Could you check a few things on this model? Use its own coordinates, in mm. A direction names the side the tool comes from. Round coordinates to 2 decimals unless told otherwise and drop trailing zeros. Write each loop counter-clockwise with the first axis right and the second up, starting at its lowest first coordinate (ties: lowest second). Pieces come first, ordered by that corner, then holes. Notation, with made-up numbers: (-7.5, 0) -> (6.5, 0) arc R18 cw to (6.5, 11) -> close; hole circle Ø4 at (-30.5, 19.5). An arc over 180 degrees is marked (long way). Answer as CSV lines item,"result". Start each with the question number.
Q1. Imagine slicing it at C-C on y = -16. Give the number of separate pieces and of enclosed holes in the cut face, and give its area (3 significant figures).
Q2. If we mould it in two halves opening along X, with no side actions, what happens to faces 4 (the cylindrical face through (68.496, -14.84, 117.029)), 5 (the flat face through (0, 96, 8)), 6 (the flat face through (55, -29, 60))? For each: pulls with the +X half, pulls with the -X half, needs draft (parallel to the pull), parting line crosses it, or undercut.
Q3. Imagine slicing it at B-B on z = 21.5. Please give me the cut outline in (x, y), and give its area (3 significant figures).
Q4. For faces 1 (the cylindrical face through (44.74, 91.85, 3.94)), 2 (the cylindrical face through (-57.093, -35.291, 4.094)), 3 (the flat face through (62.827, 24.837, 3.857)), which set-ups out of +Z, -Z, +X, -X, +Y, -Y let a thin tool reach every point of the face, with its end or its side?
Q5. Imagine slicing it at A-A on x = -5. Please give me the cut outline in (y, z), and give its area (3 significant figures).
Q6. Will these pins go through, and if not, where does the flat tip stop? pin 1 Ø8 at (x, z) = (-53, 50) entering from -Y; pin 2 Ø12 at (x, y) = (-43.5, 38.5) entering from -Z.
from build123d import *

# Parameters (mm, degrees)
F1_DEPTH      = 8
F3_DEPTH      = 70
F3_DEPTH_BACK = 70
F4_W          = 110
F4_H          = 115
F4_R          = 2
F5_DEPTH      = 10.5877977107
F6_R          = 5
F7_R          = 5


with BuildPart() as f1:
    # F0 (on Top) → F1 (new body)
    with BuildSketch(Plane.XY):
        with BuildLine():
            Line((-55.4502481405, 98.6044170713), (-70, -46.8931015238))
            Line((-70, -46.8931015238), (70, -46.8931015238))
            Line((70, -46.8931015238), (55.4502481405, 98.6044170713))
            ThreePointArc((55.4502481405, 98.6044170713), (53.8300887932, 101.8141611439), (50.4750621894, 103.1068984762))
            Line((50.4750621894, 103.1068984762), (-50.4750621894, 103.1068984762))
            ThreePointArc((-50.4750621894, 103.1068984762), (-53.8300887932, 101.8141611439), (-55.4502481405, 98.6044170713))
        make_face()
        with BuildLine():
            Line((-41.4251865683, 93.1068984762), (41.4251865683, 93.1068984762))
            ThreePointArc((41.4251865683, 93.1068984762), (44.7802131721, 91.8141611439), (46.4003725194, 88.6044170713))
            Line((46.4003725194, 88.6044170713), (58.4003725194, -31.3955829287))
            ThreePointArc((58.4003725194, -31.3955829287), (57.1324492361, -35.2481281276), (53.4251865683, -36.8931015238))
            Line((53.4251865683, -36.8931015238), (-53.4251865683, -36.8931015238))
            ThreePointArc((-53.4251865683, -36.8931015238), (-57.1324492361, -35.2481281276), (-58.4003725194, -31.3955829287))
            Line((-58.4003725194, -31.3955829287), (-46.4003725194, 88.6044170713))
            ThreePointArc((-46.4003725194, 88.6044170713), (-44.7802131721, 91.8141611439), (-41.4251865683, 93.1068984762))
        make_face(mode=Mode.SUBTRACT)
    extrude(amount=F1_DEPTH)

    # F2 (on Right) → F3 (join, two sides)
    with BuildSketch(Plane.YZ) as f3_sk:
        Polygon((-18.3058557984, 119.3901673481), (-46.8931015238, 8), (-38.633844698, 8), (-35.4294686048, 20.4858474544), (-10.5569745916, 117.4014893846), align=None)
    extrude(amount=F3_DEPTH)
    extrude(f3_sk.sketch, amount=-F3_DEPTH_BACK)

    # F4 (on face) → F5 (cut, through all)
    with BuildSketch(Plane(origin=(0, -45.9216252544, 11.7853560733), x_dir=(1, 0, 0), z_dir=(0, -0.9686101509, 0.2485847454))):
        with Locations((0, 53.5919715017)):
            Rectangle(F4_W, F4_H)
        with Locations((-62.5, 101.0919715017)):
            Circle(F4_R)
        with Locations((-62.5, 36.0919715017)):
            Circle(F4_R)
        with Locations((62.5, 36.0919715017)):
            Circle(F4_R)
        with Locations((62.5, 101.0919715017)):
            Circle(F4_R)
    extrude(amount=-F5_DEPTH, mode=Mode.SUBTRACT)

    # F6
    f6_edges = [f1.edges().sort_by_distance(p)[0] for p in [
        (-70, -14.431415, 118.395828),
        (-55, -14.431415, 118.395828),
        (55, -14.431415, 118.395828),
        (70, -14.431415, 118.395828),
    ]]
    fillet(f6_edges, radius=F6_R)

    # F7
    f7_edges = [f1.edges().sort_by_distance(p)[0] for p in [
        (-62.087037, -38.633845, 8),
        (62.087037, -38.633845, 8),
    ]]
    fillet(f7_edges, radius=F7_R)


solid = f1.part
Checks:
1,separate pieces,"4"
1,enclosed holes,"2"
1,area,"791 mm^2"
2,face 4,"pulls with the +X half"
2,face 5,"needs draft"
2,face 6,"undercut"
3,outline,"(-70, -43.43) -> (-55, -43.43) -> (-55, -35.17) -> (-70, -35.17) -> close; (55, -43.43) -> (70, -43.43) -> (70, -35.17) -> (55, -35.17) -> close"
3,area,"248 mm^2"
4,face 1,"+Z, -Z"
4,face 2,"-Z"
4,face 3,"-Z, +X, +Y"
5,outline,"(-46.89, 0) -> (-36.89, 0) -> (-36.89, 5.43) -> (-46.89, 8) -> close; (93.11, 0) -> (103.11, 0) -> (103.11, 8) -> (93.11, 8) -> close"
5,area,"147 mm^2"
6,pin 1,"y = -37"
6,pin 2,"through"
